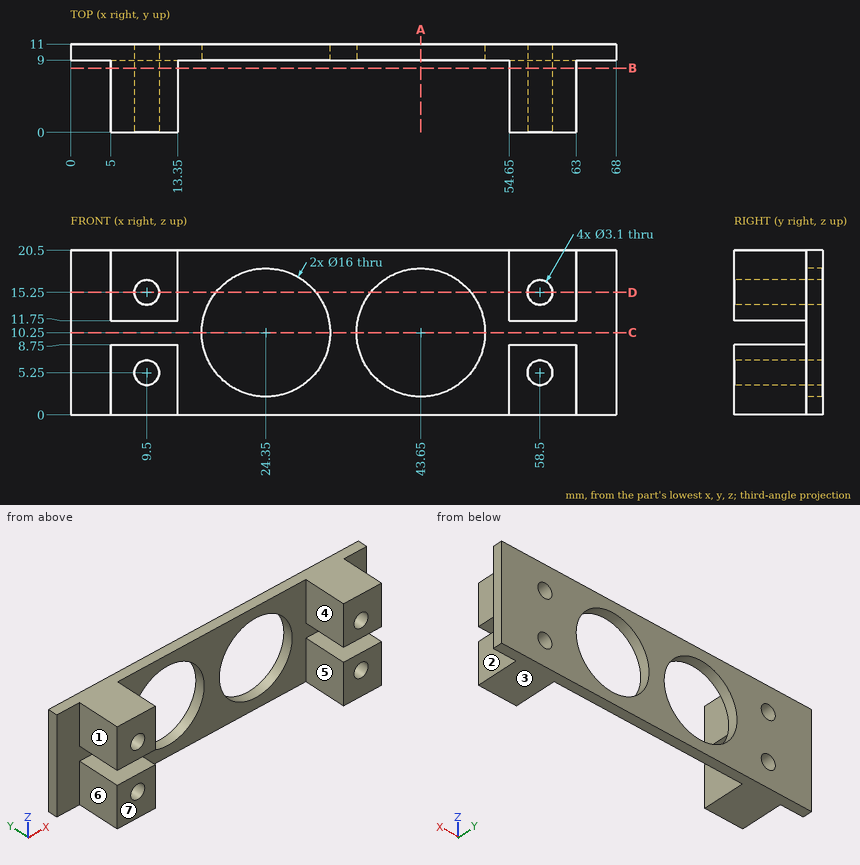
Can you work these out from the drawing? Everything is in mm from the part's minimum corner. A direction names the side the tool comes from. Coordinates: 2 decimals unless noted, no trailing zeros. Loops run counter-clockwise (first coordinate to the right, second up) from the corner with the lowest first, then second, coordinate; pieces in that order, holes last.
1) Which directions (+Z, -Z, +X, -X, +Y, -Y) give clear straight access to the entire face, cutting with the end or side of a thin tool? Please do the marked faces 5, 6 and 7.
2) Imagine slicing it at A-A on x = 43.65. List the corners of the cut face in (y, z) for me, plus the area to 3 significant figures.
3) I need wall thicknesses on probe 1 along X at (y, z) = (4.25, 5.25); probe 2 along X at (y, z) = (10.3, 10.25); probe 3 along Z at (x, y) = (58.5, 5.75). Which ranges of each line are inside material? Lowest first, please.
4) Imagine slicing it at C-C on z = 10.25. List the corners of the cut face in (x, y) for me.
5) Imagine slicing it at B-B on y = 8. List the corners of the cut face in (x, z) for me, plus the area to 3 significant figures.
6) Thinking about a two-plate mould opening in X: for the marked faces 1, 2, 3 and 4, which applies, pulls with the +X half, pulls with the -X half, needs draft (parallel to the pull), parting line crosses it, or undercut?
7) For pin 1 (3.5 mm diameter, centred on x = 9.5, z = 5.25, fed in from -Y); pin 2 (2.5 mm diameter, centred on y = 4.5, z = 18, fed in from -X); pin 3 (2.5 mm diameter, centred on y = 3, z = 15.5, fed in from +X); pin 4 (2.5 mm diameter, centred on x = 58.5, z = 15.25, fed in from +Y), each with a flat end and sliding along its axis, tell me the tip position at first contact or that it passes through.
8) Imagine slicing it at D-D on z = 15.25. List the corners of the cut face in (x, y) for me (3 decimals), plus the area to 3 significant figures.
Completed:
1. face 5: +Z, -Z, -Y
1. face 6: +Z, -Z, -X, -Y
1. face 7: +Z, -Z, +X, -X, -Y
2. outline: (9, 0) - (11, 0) - (11, 2.25) - (9, 2.25) - close; (9, 18.25) - (11, 18.25) - (11, 20.5) - (9, 20.5) - close
2. area: 9.00 mm2
3. probe 1: x = 5 to 7.95, 11.05 to 13.35, 54.65 to 56.95, 60.05 to 63
3. probe 2: x = 0 to 16.35, 32.35 to 35.65, 51.65 to 68
3. probe 3: z = 0 to 3.7, 6.8 to 8.75, 11.75 to 13.7, 16.8 to 20.5
4. outline: (0, 9) - (16.35, 9) - (16.35, 11) - (0, 11) - close; (32.35, 9) - (35.65, 9) - (35.65, 11) - (32.35, 11) - close; (51.65, 9) - (68, 9) - (68, 11) - (51.65, 11) - close
5. outline: (5, 0) - (13.35, 0) - (13.35, 8.75) - (5, 8.75) - close; (5, 11.75) - (13.35, 11.75) - (13.35, 20.5) - (5, 20.5) - close; (54.65, 0) - (63, 0) - (63, 8.75) - (54.65, 8.75) - close; (54.65, 11.75) - (63, 11.75) - (63, 20.5) - (54.65, 20.5) - close; hole circle Ø3.1 at (9.5, 5.25); hole circle Ø3.1 at (9.5, 15.25); hole circle Ø3.1 at (58.5, 5.25); hole circle Ø3.1 at (58.5, 15.25)
5. area: 262 mm2
6. face 1: pulls with the -X half
6. face 2: pulls with the +X half
6. face 3: needs draft
6. face 4: undercut
7. pin 1: stops at y = 0
7. pin 2: stops at x = 5
7. pin 3: stops at x = 63
7. pin 4: passes through
8. outline: (0, 9) - (5, 9) - (5, 0) - (7.95, 0) - (7.95, 11) - (0, 11) - close; (11.05, 0) - (13.35, 0) - (13.35, 9) - (18.105, 9) - (18.105, 11) - (11.05, 11) - close; (30.595, 9) - (37.405, 9) - (37.405, 11) - (30.595, 11) - close; (49.895, 9) - (54.65, 9) - (54.65, 0) - (56.95, 0) - (56.95, 11) - (49.895, 11) - close; (60.05, 0) - (63, 0) - (63, 9) - (68, 9) - (68, 11) - (60.05, 11) - close
8. area: 168 mm2
